from build123d import *

# Parameters (mm, degrees)
SKETCH_1_W            = 50
SKETCH_1_H            = 7
EXTRUDE_1_DEPTH       = 22
HOLE_WIZARD_M31_D     = 3.15
HOLE_WIZARD_M31_DEPTH = 10
HOLE_WIZARD_M31_TIP   = 0.946355475
HOLE_WIZARD_M32_D     = 3.15
HOLE_WIZARD_M32_DEPTH = 10
HOLE_WIZARD_M32_TIP   = 0.946355475


with BuildPart() as part:
    # Эскиз1 → Бобышка-Вытянуть1 (new body)
    with BuildSketch(Plane(origin=(0, 0, 0), x_dir=(0, 0, -1), z_dir=(1, 0, 0))):
        with Locations((-20.27623422, 0.143640104)):
            Rectangle(SKETCH_1_W, SKETCH_1_H)
    extrude(amount=EXTRUDE_1_DEPTH)

    # Сверло под метчик  спиральное M31
    with Locations(Plane(origin=(22, 0, 0), x_dir=(0, 0, -1), z_dir=(1, 0, 0))):
        with Locations((-35.27623422, 0.143640104), (-5.27623422, 0.143640104)):
            Hole(HOLE_WIZARD_M31_D / 2, depth=HOLE_WIZARD_M31_DEPTH)
            with Locations((0, 0, -(HOLE_WIZARD_M31_DEPTH + HOLE_WIZARD_M31_TIP / 2))):  # 118° drill point
                Cone(0, HOLE_WIZARD_M31_D / 2, HOLE_WIZARD_M31_TIP, mode=Mode.SUBTRACT)

    # Сверло под метчик  спиральное M32
    with Locations(Plane.ZY):
        with Locations((20.27623422, 0.143640104)):
            Hole(HOLE_WIZARD_M32_D / 2, depth=HOLE_WIZARD_M32_DEPTH)
            with Locations((0, 0, -(HOLE_WIZARD_M32_DEPTH + HOLE_WIZARD_M32_TIP / 2))):  # 118° drill point
                Cone(0, HOLE_WIZARD_M32_D / 2, HOLE_WIZARD_M32_TIP, mode=Mode.SUBTRACT)


solid = part.part
Source: CAD feature listing. Evaluate the final solid. Frame: model axes, mm. A direction names the side the tool comes from. Coordinates: 2 decimals unless noted, no trailing zeros. Order: outer loops, then holes, each group sorted by start corner. A loop starts at its lowest first (then second) coordinate and runs counter-clockwise, first axis right, second up.
Item 1: Cut plane B-B (x = 14.5). Return loops of the section in (y, z) (3 decimals).
Output values:
outline: (-3.356, -4.724) - (3.644, -4.724) - (3.644, 45.276) - (-3.356, 45.276) - close; hole circle Ø3.15 at (0.144, 5.276); hole circle Ø3.15 at (0.144, 35.276)
Item 2: Pull-direction query (Y, two-part tool) for faces 1 (the face through (22, 0, 21)), 2 (the face through (11, 3.644, 21)), 3 (the face through (11, -3.356, 21)), 4 (the face through (11.22, 0.16, 35.55)); classes: pulls with the +Y half, pulls with the -Y half, needs draft (parallel to the pull), parting line crosses it, or undercut.
Output values:
face 1: needs draft
face 2: pulls with the +Y half
face 3: pulls with the -Y half
face 4: undercut
Item 3: First-contact query: P1, Ø2.5, axis at y = 0.14, z = 5.28, coming from the +X side. Flat tip, straight axial feed; report the tip coordinate or a pass-through.
Output values:
P1: stops at x = 11.81
Item 4: Set-up query: faces 5 (the face through (5.07, 0.617, 18.774)), 6 (the face through (11, 0, -4.724)), 7 (the face through (16.93, 0.617, 6.779)). Return all of +Z, -Z, +X, -X, +Y, -Y with unobstructed straight access to the full face (end or side cutting, diameter ignored); none if empty.
Output values:
face 5: -X
face 6: -Z, +X, -X, +Y, -Y
face 7: +X
Item 5: Material intervals for line 1 (Z direction, x = 21, y = 0); line 2 (Z direction, x = 20, y = -0.75); line 3 (Z direction, x = 1.25, y = -1), sorted ascending.
Output values:
line 1: z = -4.72 to 3.71, 6.84 to 33.71, 36.84 to 45.28
line 2: z = -4.72 to 3.98, 6.57 to 33.98, 36.57 to 45.28
line 3: z = -4.72 to 19.19, 21.36 to 45.28
Item 6: Cut plane A-A (x = 8). Return loops of the section in (y, z) (3 decimals), plus the area to 3 significant figures.
Output values:
outline: (-3.356, -4.724) - (3.644, -4.724) - (3.644, 45.276) - (-3.356, 45.276) - close; hole circle Ø3.15 at (0.144, 20.276)
area: 342 mm2
